```python
from build123d import *

# Parameters (mm, degrees)
BOSS_EXTRUDE1_DEPTH = 1
BOSS_EXTRUDE2_DEPTH = 37
SKETCH4_W           = 76
SKETCH4_H           = 10
BOSS_EXTRUDE3_DEPTH = 0.5


with BuildPart() as part:
    # Sketch1 → Boss-Extrude1 (new body)
    with BuildSketch(Plane(origin=(0, 0, 0), x_dir=(0, 0, -1), z_dir=(1, 0, 0))):
        Polygon((-39, 10.5), (-38, 10.5), (-38, 3.5), (-26.539616882, 3.5), (-19.376877433, -1.5), (19.376877433, -1.5), (26.539616882, 3.5), (38, 3.5), (38, 10.5), (39, 10.5), (39, -10.5), (-39, -10.5), align=None)
    boss_extrude1 = extrude(amount=BOSS_EXTRUDE1_DEPTH)

    # Sketch2 → Boss-Extrude2 (add)
    with BuildSketch(Plane(origin=(1, 0, 0), x_dir=(0, 0, -1), z_dir=(1, 0, 0))):
        Polygon((-38, 10.5), (-38, -9.5), (38, -9.5), (38, 10.5), (39, 10.5), (39, -10.5), (-39, -10.5), (-39, 10.5), align=None)
    extrude(amount=BOSS_EXTRUDE2_DEPTH)

    # Mirror1: Boss-Extrude1 across plane
    add(boss_extrude1.mirror(Plane(origin=(19.5, 0, 0), x_dir=(0, 0, 1), z_dir=(1, 0, 0))))

    # Sketch4 → Boss-Extrude3 (add, symmetric)
    with BuildSketch(Plane(origin=(19.5, 0, 0), x_dir=(0, 0, -1), z_dir=(1, 0, 0))):
        with Locations((0, -4.5)):
            Rectangle(SKETCH4_W, SKETCH4_H)
    extrude(amount=BOSS_EXTRUDE3_DEPTH, both=True)


solid = part.part
```
The listing builds one solid part. Answer for the finished solid, in the listing's coordinates (mm). A direction names the side the tool comes from. Give positions to 0.01 mm unless a question says otherwise; leave off trailing zeros. Order: outer loops, then holes, each group sorted by start corner. A loop starts at its lowest first (then second) coordinate and runs counter-clockwise, first axis right, second up. Notation, with made-up numbers: M 17.5,58 L 42.5,58 A29 ccw 42.5,82 Z; hole C 13.25,73 d8. An arc over 180 degrees is marked long. Put each result on its own line as item: value. Start each with the question number.
Item 1: Which of the six approach directions +Z, -Z, +X, -X, +Y, -Y give full straight-line access (tool end or side, diameter ignored) to faces 1 (the face through (20, -10.5, -1)), 2 (the face through (0.493, 1.035, 23.008)), 3 (the face through (20, 3, -38)), 4 (the face through (38.507, 1.035, 23.008)), 5 (the face through (39, -5, -1))?
Item 2: For a pull along Z with two mould halves and no side action, classify faces 6 (the face through (20, 0, 39)), 7 (the face through (0, -5, -1)), 8 (the face through (20, -4, 1)) as +Z half, -Z half, draft (parallel to the pull), parting line (faces both ways), or undercut.
Item 3: The part is cut by section B-B, the plane y = 4.25. Determine the outline of the cut face in (x, z), and give its area (3 significant figures).
Item 4: The part is cut by section A-A, the plane y = -8.75. Determine the outline of the cut face in (x, z), and give its area (3 significant figures).
Item 5: Flat-ended cylindrical pins translate along their axes: P1, Ø8, axis at y = -2.5, z = -17.5, coming from the -X side; P2, Ø4, axis at x = 9.5, z = 19, coming from the +Y side; P3, Ø14.5, axis at x = 6.5, z = -3, coming from the +Y side; P4, Ø0.8, axis at x = 38.5, z = 30, coming from the +Y side. Find the tip coordinate at first contact, or state that the pin passes through.
Item 6: The part is cut by section D-D, the plane x = 11.5. Determine the outline of the cut face in (y, z), and give its area (3 significant figures).
Item 7: Find the intervals of material crossed by line 1 along X through (y, z) = (-0.5, 29.5); line 2 along Z through (x, y) = (9.5, 3.75); line 3 along Y through (x, z) = (28.5, -20), in increasing order.
Item 8: The part is cut by section C-C, the plane z = -11.5. Determine the outline of the cut face in (x, y), and give its area (3 significant figures).
Answer key:
1. face 1: +Z, -Z, +X, -X, -Y
1. face 2: -X, +Y
1. face 3: +Y
1. face 4: +X, +Y
1. face 5: +Z, -Z, +X, +Y, -Y
2. face 6: +Z half
2. face 7: draft
2. face 8: undercut
3. outline: M 0,-39 L 39,-39 L 39,-38 L 0,-38 Z; M 0,38 L 39,38 L 39,39 L 0,39 Z
3. area: 78.0 mm²
4. outline: M 0,-39 L 39,-39 L 39,39 L 0,39 Z; hole M 1,-38 L 19,-38 L 19,38 L 1,38 Z; hole M 20,-38 L 38,-38 L 38,38 L 20,38 Z
4. area: 306 mm²
5. P1: stops at x = 0
5. P2: stops at y = -9.5
5. P3: stops at y = -1.5
5. P4: stops at y = 3.5
6. outline: M -10.5,-39 L 10.5,-39 L 10.5,-38 L -9.5,-38 L -9.5,38 L 10.5,38 L 10.5,39 L -10.5,39 Z
6. area: 118 mm²
7. line 1: x = 0 to 1, 19 to 20, 38 to 39
7. line 2: z = -39 to -38, 38 to 39
7. line 3: y = -10.5 to -9.5
8. outline: M 0,-10.5 L 39,-10.5 L 39,-1.5 L 38,-1.5 L 38,-9.5 L 20,-9.5 L 20,0.5 L 19,0.5 L 19,-9.5 L 1,-9.5 L 1,-1.5 L 0,-1.5 Z
8. area: 65.0 mm²
